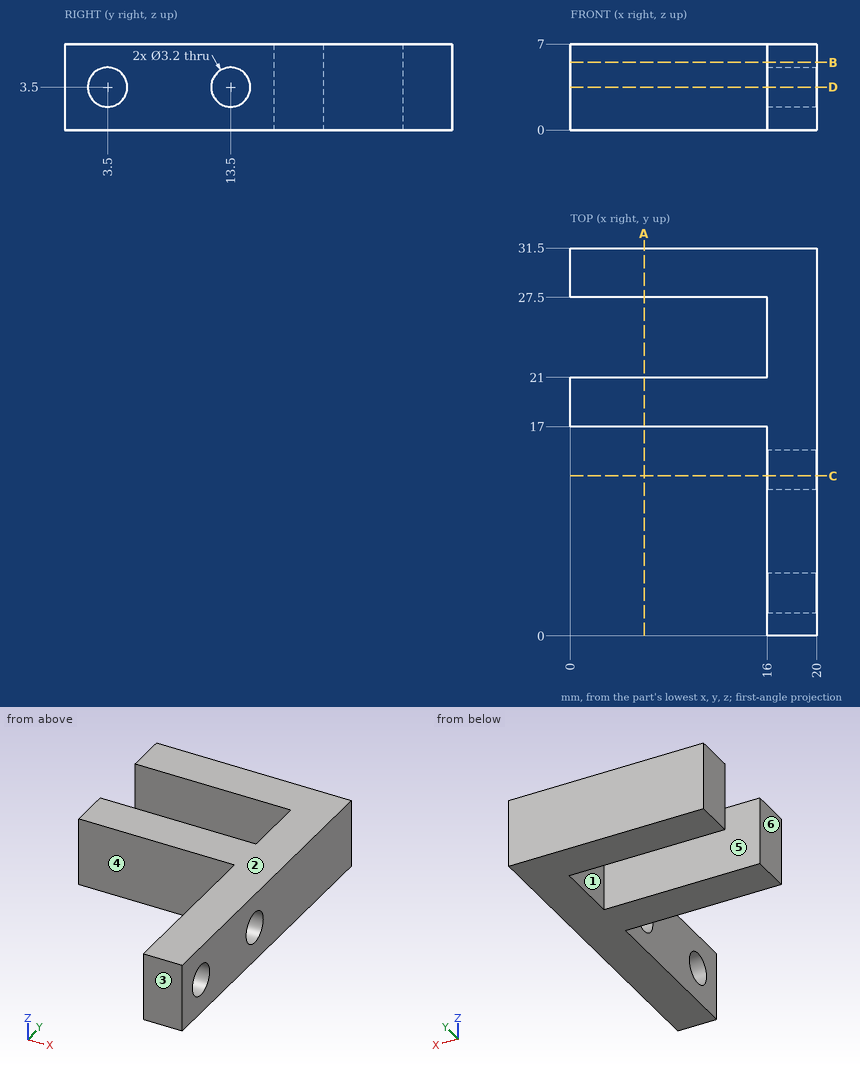
Study the drawing (mm; zero at the part's minimum x, y, z) and answer. A direction names the side the tool comes from. Coordinates: 2 decimals unless noted, no trailing zeros. Loops run counter-clockwise (first coordinate to the right, second up) from the corner with the lowest first, then second, coordinate; pieces in that order, holes last. Notation, with made-up numbers: (18, -33) -> (76, -33) arc R21 ccw to (76, -27) -> close; hole circle Ø6 at (17, 10). An arc over 180 degrees is marked (long way). Write item = value, one per line. Start each with the question number.
1) For the marked faces 4, 5 and 6, determine the directions among +Z, -Z, +X, -X, +Y, -Y from which every point of the face is accessible in a straight line to the end or side of a thin tool.
2) The part is cut by section C-C, the plane y = 13. Determine the outline of the cut face in (x, z), plus the area to 3 significant figures.
3) The mould has two halves that part along Y. Classify the marked faces 1, 2 and 3: pulls with the +Y half, pulls with the -Y half, needs draft (parallel to the pull), parting line crosses it, or undercut.
4) The part is cut by section D-D, the plane z = 3.5. Determine the outline of the cut face in (x, y), plus the area to 3 significant figures.
5) The part is cut by section B-B, the plane z = 5.5. Determine the outline of the cut face in (x, y).
6) The part is cut by section A-A, the plane x = 6. Determine the outline of the cut face in (y, z), plus the area to 3 significant figures.
7) Given P1, Ø3.5, axis at x = 6, z = 5, coming from the -Y side; P2, Ø3.5, axis at y = 9, z = 3.5, coming from the -X side, each flat-ended and moving along its own axis, determine where each tip first touches the part or whether it passes through.
8) Find the intervals of material crossed by L1, parallel to Y at x = 14, z = 5; L2, parallel to Z at x = 18.3, y = 13.5; L3, parallel to X at y = 9, z = 3, in increasing order. Write a range as from..to.
Result:
q1.face_4 = +Z, -Z, -X, -Y
q1.face_5 = +Z, -Z, -X
q1.face_6 = +Z, -Z, -X, +Y, -Y
q2.outline = (16, 0) -> (20, 0) -> (20, 1.98) -> (16, 1.98) -> close; (16, 5.02) -> (20, 5.02) -> (20, 7) -> (16, 7) -> close
q2.area = 15.8 mm²
q3.face_1 = undercut
q3.face_2 = needs draft
q3.face_3 = pulls with the -Y half
q4.outline = (0, 17) -> (16, 17) -> (16, 15.1) -> (20, 15.1) -> (20, 31.5) -> (0, 31.5) -> (0, 27.5) -> (16, 27.5) -> (16, 21) -> (0, 21) -> close; (16, 0) -> (20, 0) -> (20, 1.9) -> (16, 1.9) -> close; (16, 5.1) -> (20, 5.1) -> (20, 11.9) -> (16, 11.9) -> close
q4.area = 228 mm²
q5.outline = (0, 17) -> (16, 17) -> (16, 0) -> (20, 0) -> (20, 31.5) -> (0, 31.5) -> (0, 27.5) -> (16, 27.5) -> (16, 21) -> (0, 21) -> close
q6.outline = (17, 0) -> (21, 0) -> (21, 7) -> (17, 7) -> close; (27.5, 0) -> (31.5, 0) -> (31.5, 7) -> (27.5, 7) -> close
q6.area = 56.0 mm²
q7.P1 = 17
q7.P2 = 16
q8.L1 = 17..21, 27.5..31.5
q8.L2 = 0..1.9, 5.1..7
q8.L3 = 16..20
